For this review, take the finished solid that the model builds, in its own axes (mm). Round coordinates to 2 decimals unless told otherwise and drop trailing zeros. Write each loop counter-clockwise with the first axis right and the second up, starting at its lowest first coordinate (ties: lowest second). Pieces come first, ordered by that corner, then holes. Notation, with made-up numbers: (-4.5, -21.75) -> (50.5, -21.75) arc R10 cw to (50.5, -7.75) -> close; hole circle Ø4 at (38.25, -30). An arc over 180 degrees is marked (long way). Write each question's results on one line, items separated by ' | '. Start each with the question number.
Item 1: The part is to be moulded in two halves that separate along Z. For faces 1 (the flat face through (76, -9, 371)), 2 (the flat face through (559, -16, 308)), say which applies: +Z half, -Z half, draft (parallel to the pull), parting line (faces both ways), or undercut.
Item 2: To check wall thickness, follow line 1 along X through (y, z) = (-12.5, 130.5); line 2 along Z through (x, y) = (432.5, -10.25); line 3 along X through (y, z) = (-13.5, 335). State the ranges of each line that lie inside material, in increasing order.
Item 3: Add section D-D (z = 648). State the section outline as (x, y) points.
Item 4: Add section B-B (z = 737). State the section outline as (x, y) points.
Item 5: Add section C-C (x = 245). State the section outline as (y, z) points.
Item 6: Add section A-A (x = 530). State the section outline as (y, z) points.
from build123d import *

# Parameters (mm, degrees)
F0_W      = 44.656470418
F0_H      = 33.8078811765
F1_DEPTH  = 16
F2_DEPTH  = 796
F3_DEPTH  = 196
F4_W      = 68.9578056335
F4_H      = 493.6993122101
F5_DEPTH  = 7
F6_DEPTH  = 9.7
F7_DEPTH  = 99.33
F8_DEPTH  = 99.33
F9_DEPTH  = 17.34
F10_DEPTH = 102.97
F11_W     = 35.2807044983
F11_H     = 492.0964837074
F12_DEPTH = 7
F13_DEPTH = 37.27
F14_DEPTH = 6.58
F15_DEPTH = 106.63
F16_DEPTH = 5.87
F17_DEPTH = 200
F18_DEPTH = 200
F19_DEPTH = 200
F20_DEPTH = 200
F21_DEPTH = 200
F22_DEPTH = 200
F23_R     = 3


with BuildPart() as f1:
    # F0 (on Front) → F1 (new body)
    with BuildSketch(Plane.XZ):
        with Locations((22.328235209, 16.9039405882)):
            Rectangle(F0_W, F0_H)
    extrude(amount=F1_DEPTH)

    # F2 (add): a face of the model
    f2_faces = [f1.faces().sort_by_distance(p)[0] for p in [
        (22.328235209, -8, 0),
    ]]
    extrude(f2_faces, amount=-F2_DEPTH)

    # F3 (add): a face of the model
    f3_faces = [f1.faces().sort_by_distance(p)[0] for p in [
        (0, -8, 398),
    ]]
    extrude(f3_faces, amount=-F3_DEPTH)

    # F4 (on face) → F5 (cut)
    with BuildSketch(Plane.XZ.offset(16)):
        with Locations((94.1769480705, 399.8196721077)):
            Rectangle(F4_W, F4_H)
    extrude(amount=-F5_DEPTH, mode=Mode.SUBTRACT)

    # F6 (cut): a face of the model
    f6_faces = [f1.faces().sort_by_distance(p)[0] for p in [
        (59.6980452538, -12.5, 399.8196721077),
    ]]
    extrude(f6_faces, amount=-F6_DEPTH, mode=Mode.SUBTRACT)

    # F7 (add): a face of the model
    f7_faces = [f1.faces().sort_by_distance(p)[0] for p in [
        (89.3269480705, -12.5, 646.6693282127),
    ]]
    extrude(f7_faces, amount=-F7_DEPTH)

    # F8 (cut): a face of the model
    f8_faces = [f1.faces().sort_by_distance(p)[0] for p in [
        (89.3269480705, -12.5, 646.6693282127),
    ]]
    extrude(f8_faces, amount=-F8_DEPTH, mode=Mode.SUBTRACT)

    # F9 (cut): a face of the model
    f9_faces = [f1.faces().sort_by_distance(p)[0] for p in [
        (128.6558508873, -12.5, 449.4846721077),
    ]]
    extrude(f9_faces, amount=-F9_DEPTH, mode=Mode.SUBTRACT)

    # F10 (cut): a face of the model
    f10_faces = [f1.faces().sort_by_distance(p)[0] for p in [
        (97.9969480705, -12.5, 152.9700160027),
    ]]
    extrude(f10_faces, amount=-F10_DEPTH, mode=Mode.SUBTRACT)

    # F11 (on face) → F12 (join)
    with BuildSketch(Plane.XZ.offset(9)):
        with Locations((91.7714834213, 432.6795041561)):
            Rectangle(F11_W, F11_H)
    extrude(amount=F12_DEPTH)

    # F13 (add): a face of the model
    f13_faces = [f1.faces().sort_by_distance(p)[0] for p in [
        (91.7714834213, -12.5, 678.7277460098),
    ]]
    extrude(f13_faces, amount=F13_DEPTH)

    # F14 (add): a face of the model
    f14_faces = [f1.faces().sort_by_distance(p)[0] for p in [
        (109.4118356705, -12.5, 451.3145041561),
    ]]
    extrude(f14_faces, amount=F14_DEPTH)

    # F15 (add): a face of the model
    f15_faces = [f1.faces().sort_by_distance(p)[0] for p in [
        (95.0614834213, -12.5, 186.6312623024),
    ]]
    extrude(f15_faces, amount=F15_DEPTH)

    # F16 (cut): a face of the model
    f16_faces = [f1.faces().sort_by_distance(p)[0] for p in [
        (74.1311311722, -12.5, 397.9995041561),
    ]]
    extrude(f16_faces, amount=-F16_DEPTH, mode=Mode.SUBTRACT)

    # F17 (add): a face of the model
    f17_faces = [f1.faces().sort_by_distance(p)[0] for p in [
        (196, -8, 398),
    ]]
    extrude(f17_faces, amount=F17_DEPTH)

    # F18 (cut): a face of the model
    f18_faces = [f1.faces().sort_by_distance(p)[0] for p in [
        (145.9958508873, -12.5, 397.9996721077),
    ]]
    extrude(f18_faces, amount=-F18_DEPTH, mode=Mode.SUBTRACT)

    # F19 (add): a face of the model
    f19_faces = [f1.faces().sort_by_distance(p)[0] for p in [
        (115.9918356705, -12.5, 397.9995041561),
    ]]
    extrude(f19_faces, amount=F19_DEPTH)

    # F20 (add): a face of the model
    f20_faces = [f1.faces().sort_by_distance(p)[0] for p in [
        (396, -8, 398),
    ]]
    extrude(f20_faces, amount=F20_DEPTH)

    # F21 (cut): a face of the model
    f21_faces = [f1.faces().sort_by_distance(p)[0] for p in [
        (345.9958508873, -12.5, 397.9996721077),
    ]]
    extrude(f21_faces, amount=-F21_DEPTH, mode=Mode.SUBTRACT)

    # F22 (add): a face of the model
    f22_faces = [f1.faces().sort_by_distance(p)[0] for p in [
        (315.9918356705, -12.5, 397.9995041561),
    ]]
    extrude(f22_faces, amount=F22_DEPTH)

    # F23
    f23_edges = [f1.edges().sort_by_distance(p)[0] for p in [
        (297.996483, -16, 715.997746),
        (80.001131, -16, 397.999504),
        (297.996483, -16, 80.001262),
        (515.991836, -16, 397.999504),
        (0, -16, 398),
        (298, -16, 0),
        (596, -16, 398),
        (298, -16, 796),
        (49.998045, -16, 397.999672),
        (297.996948, -16, 745.999328),
        (545.995851, -16, 397.999672),
        (297.996948, -16, 50.000016),
    ]]
    fillet(f23_edges, radius=F23_R)


solid = f1.part
Responses:
1) face 1: undercut | face 2: draft
2) line 1: x = 0 to 50, 80 to 515.99, 546 to 596 | line 2: z = 0 to 50, 80 to 716, 746 to 796 | line 3: x = 0.04 to 49.96, 80.04 to 515.95, 546.04 to 595.96
3) outline: (0, -13) arc R3 ccw to (3, -16) -> (47, -16) arc R3 ccw to (50, -13) -> (50, -9) -> (80, -9) -> (80, -13) arc R3 ccw to (83, -16) -> (512.99, -16) arc R3 ccw to (515.99, -13) -> (515.99, -9) -> (546, -9) -> (546, -13) arc R3 ccw to (549, -16) -> (593, -16) arc R3 ccw to (596, -13) -> (596, 0) -> (0, 0) -> close
4) outline: (0, -13) arc R3 ccw to (3, -16) -> (47, -16) arc R3 ccw to (50, -13) -> (50, -9) -> (546, -9) -> (546, -13) arc R3 ccw to (549, -16) -> (593, -16) arc R3 ccw to (596, -13) -> (596, 0) -> (0, 0) -> close
5) outline: (-16, 3) arc R3 ccw to (-13, 0) -> (0, 0) -> (0, 796) -> (-13, 796) arc R3 ccw to (-16, 793) -> (-16, 749) arc R3 ccw to (-13, 746) -> (-9, 746) -> (-9, 716) -> (-13, 716) arc R3 ccw to (-16, 713) -> (-16, 83) arc R3 ccw to (-13, 80) -> (-9, 80) -> (-9, 50) -> (-13, 50) arc R3 ccw to (-16, 47) -> close
6) outline: (-16, 3) arc R3 ccw to (-13, 0) -> (0, 0) -> (0, 796) -> (-13, 796) arc R3 ccw to (-16, 793) -> (-16, 749) arc R3 ccw to (-13, 746) -> (-9, 746) -> (-9, 50) -> (-13, 50) arc R3 ccw to (-16, 47) -> close
